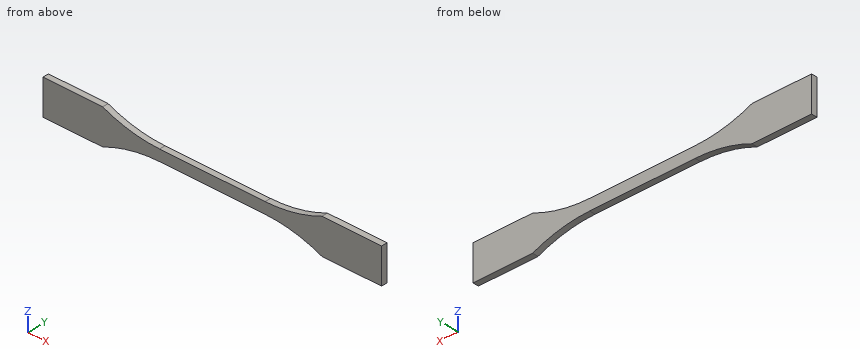
from build123d import *

# Parameters (mm, degrees)
CROQUIS1_W              = 57
CROQUIS1_H              = 6
SALIENTE_EXTRUIR1_DEPTH = 1.6


with BuildPart() as part:
    # Croquis1 → Saliente-Extruir1 (new body, symmetric)
    with BuildSketch(Plane(origin=(0, 0, 0), x_dir=(1, 0, 0), z_dir=(0, 1, 0))):
        with BuildLine():
            Line((-91.5, -9.5), (-59.253048629, -9.5))
            ThreePointArc((-59.253048629, -9.5), (-44.216233646, -4.64275422), (-28.5, -3))
            Line((-28.5, -3), (-28.5, 3))
            ThreePointArc((-28.5, 3), (-44.216233646, 4.64275422), (-59.253048629, 9.5))
            Line((-59.253048629, 9.5), (-91.5, 9.5))
            Line((-91.5, 9.5), (-91.5, -9.5))
        make_face()
        with BuildLine():
            Line((59.253048629, -9.5), (91.5, -9.5))
            Line((91.5, -9.5), (91.5, 9.5))
            Line((91.5, 9.5), (59.253048629, 9.5))
            ThreePointArc((59.253048629, 9.5), (44.216233646, 4.64275422), (28.5, 3))
            Line((28.5, 3), (28.5, -3))
            ThreePointArc((28.5, -3), (44.216233646, -4.64275422), (59.253048629, -9.5))
        make_face()
        Rectangle(CROQUIS1_W, CROQUIS1_H)
    extrude(amount=SALIENTE_EXTRUIR1_DEPTH, both=True)


solid = part.part
Source: CAD feature listing. Evaluate the final solid. Frame: model axes, mm. Round coordinates to 2 decimals unless told otherwise and drop trailing zeros. Loops run counter-clockwise (first coordinate to the right, second up) from the corner with the lowest first, then second, coordinate; pieces in that order, holes last.
Q1. Section C-C, the plane z = -5.75. Return loops of the section in (x, y), plus the area to 3 significant figures.
Q2. Section D-D, the plane x = 43.5. Return loops of the section in (y, z), plus the area to 3 significant figures.
Q3. Ray query, line 1 (Z direction, x = 10, y = 1.4); line 2 (Z direction, x = -55.5, y = 0.2). Return the intervals inside material, ascending.
Q4. First-contact query: P1, Ø1.6, axis at x = 6, y = 0.5, coming from the -Z side. Flat tip, straight axial feed; report the tip coordinate or a pass-through.
Q5. Section B-B, the plane y = 0.1. Return loops of the section in (x, z).
Q6. Section A-A, the plane z = 5.25. Return loops of the section in (x, y), plus the area to 3 significant figures.
Solutions:
1. outline: (-91.5, -1.6) - (-48.76, -1.6) - (-48.76, 1.6) - (-91.5, 1.6) - close; (48.76, -1.6) - (91.5, -1.6) - (91.5, 1.6) - (48.76, 1.6) - close
1. area: 274 mm2
2. outline: (-1.6, -4.49) - (1.6, -4.49) - (1.6, 4.49) - (-1.6, 4.49) - close
2. area: 28.8 mm2
3. line 1: z = -3 to 3
3. line 2: z = -7.96 to 7.96
4. P1: stops at z = -3
5. outline: (-91.5, -9.5) - (-59.25, -9.5) arc R76 cw to (-28.5, -3) - (28.5, -3) arc R76 cw to (59.25, -9.5) - (91.5, -9.5) - (91.5, 9.5) - (59.25, 9.5) arc R76 cw to (28.5, 3) - (-28.5, 3) arc R76 cw to (-59.25, 9.5) - (-91.5, 9.5) - close
6. outline: (-91.5, -1.6) - (-46.86, -1.6) - (-46.86, 1.6) - (-91.5, 1.6) - close; (46.86, -1.6) - (91.5, -1.6) - (91.5, 1.6) - (46.86, 1.6) - close
6. area: 286 mm2
